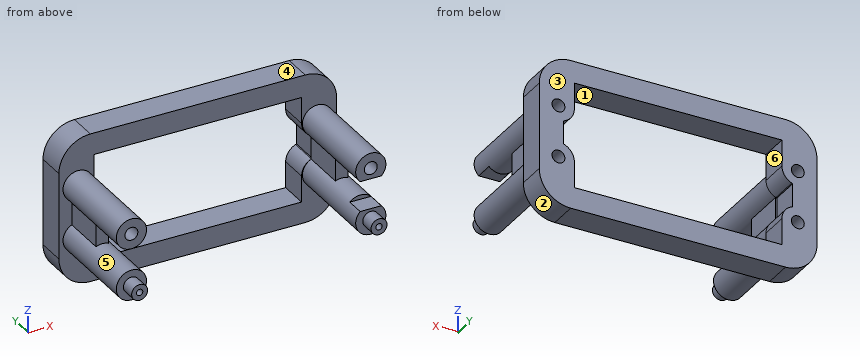
from build123d import *

# Parameters (mm, degrees)
SKETCH1_R           = 3.048
SKETCH1_R_2         = 1.2319
BOSS_EXTRUDE1_DEPTH = 25.4
SKETCH2_W           = 56.0832
SKETCH2_H           = 30.1244
BOSS_EXTRUDE3_DEPTH = 5.842
FILLET1_R           = 3.175
FILLET3_R           = 6.35
SKETCH6_W           = 5.842
SKETCH6_H           = 8.89
BOSS_EXTRUDE4_DEPTH = 1.27
SKETCH7_W           = 5.842
SKETCH7_H           = 8.89
BOSS_EXTRUDE5_DEPTH = 1.27
SKETCH16_R          = 1.6129
BOSS_EXTRUDE6_DEPTH = 3.0226
SKETCH19_R          = 1.30175
CUT_EXTRUDE1_DEPTH  = 63.809652383
SKETCH20_R          = 1.30175
CUT_EXTRUDE2_DEPTH  = 63.809652383
BOSS_EXTRUDE7_START = -12.3825
SKETCH21_R          = 1.30175
SKETCH21_R_2        = 0.635
BOSS_EXTRUDE7_DEPTH = 12.3825
SKETCH24_W          = 6.93711536
SKETCH24_H          = 6.096
CUT_EXTRUDE4_DEPTH  = 3.81


with BuildPart() as part:
    # Sketch1 → Boss-Extrude1 (new body)
    # profile 1 of 8: a face of its own
    with BuildSketch(Plane(origin=(0, 0, 0), x_dir=(1, 0, 0), z_dir=(0, 1, 0))):
        with Locations(Location((0, -10.4394, 0), (0, 0, 270))):
            Circle(SKETCH1_R)
        with Locations((0, -10.4394)):
            Circle(SKETCH1_R_2, mode=Mode.SUBTRACT)
    # profile 2 of 8: a face of its own
    with BuildSketch(Plane(origin=(0, 0, 0), x_dir=(1, 0, 0), z_dir=(0, 1, 0))):
        with Locations((0, -10.4394)):
            Circle(SKETCH1_R_2)
    # profile 3 of 8: a face of its own
    with BuildSketch(Plane(origin=(0, 0, 0), x_dir=(1, 0, 0), z_dir=(0, 1, 0))):
        with Locations(Location((0, 0, 0), (0, 0, 270))):
            Circle(SKETCH1_R)
        Circle(SKETCH1_R_2, mode=Mode.SUBTRACT)
    # profile 4 of 8: a face of its own
    with BuildSketch(Plane(origin=(0, 0, 0), x_dir=(1, 0, 0), z_dir=(0, 1, 0))):
        Circle(SKETCH1_R_2)
    # profile 5 of 8: a face of its own
    with BuildSketch(Plane(origin=(0, 0, 0), x_dir=(1, 0, 0), z_dir=(0, 1, 0))):
        with Locations(Location((-48.3362, -10.4394, 0), (0, 0, 270))):
            Circle(SKETCH1_R)
        with Locations((-48.3362, -10.4394)):
            Circle(SKETCH1_R_2, mode=Mode.SUBTRACT)
    # profile 6 of 8: a face of its own
    with BuildSketch(Plane(origin=(0, 0, 0), x_dir=(1, 0, 0), z_dir=(0, 1, 0))):
        with Locations((-48.3362, -10.4394)):
            Circle(SKETCH1_R_2)
    # profile 7 of 8: a face of its own
    with BuildSketch(Plane(origin=(0, 0, 0), x_dir=(1, 0, 0), z_dir=(0, 1, 0))):
        with Locations(Location((-48.3362, 0, 0), (0, 0, 270))):
            Circle(SKETCH1_R)
        with Locations((-48.3362, 0)):
            Circle(SKETCH1_R_2, mode=Mode.SUBTRACT)
    # profile 8 of 8: a face of its own
    with BuildSketch(Plane(origin=(0, 0, 0), x_dir=(1, 0, 0), z_dir=(0, 1, 0))):
        with Locations((-48.3362, 0)):
            Circle(SKETCH1_R_2)
    extrude(amount=-BOSS_EXTRUDE1_DEPTH)

    # Sketch2 → Boss-Extrude3 (add)
    with BuildSketch(Plane(origin=(0, 0, 0), x_dir=(1, 0, 0), z_dir=(0, 1, 0))):
        with Locations((-24.1681, -5.2197)):
            Rectangle(SKETCH2_W, SKETCH2_H)
        Polygon((-47.3075, -2.794), (-45.1231, -2.794), (-45.1231, 5.4483), (-3.2131, 5.4483), (-3.2131, -2.794), (-1.0287, -2.794), (-1.0287, -7.6454), (-3.2131, -7.6454), (-3.2131, -15.8877), (-45.1231, -15.8877), (-45.1231, -7.6454), (-47.3075, -7.6454), align=None, mode=Mode.SUBTRACT)
    extrude(amount=-BOSS_EXTRUDE3_DEPTH)

    # Fillet1
    # the kernel refuses this fillet: 3.175 mm, written as the material it takes off along each edge
    with BuildSketch(Plane(origin=(-3.2131, 7.368907547, 7.6454), x_dir=(1, 0, 0), z_dir=(0, -1, 0)), Plane(origin=(-45.1231, 7.368907547, 2.794), x_dir=(-1, 0, 0), z_dir=(0, -1, 0))) as fillet1_piece_1:
        with BuildLine():
            CenterArc((3.175, 2.947563019), FILLET1_R, 180, 68.181567229)
            Line((0, 2.947563019), (-0.0635, 2.947563019))
            Line((-0.0635, 2.947563019), (-0.0635, 0))
            Line((-0.0635, 0), (0, -0.0635))
            ThreePointArc((0, -0.0635), (0.997479397, -0.0635), (1.971357969, -0.05895126))
            Line((1.971357969, -0.05895126), (1.994958793, 0))
        make_face()
    extrude(amount=20.579815094, mode=Mode.SUBTRACT)
    with BuildSketch(Plane(origin=(-3.2131, 7.368907547, 2.794), x_dir=(0, 0, -1), z_dir=(0, -1, 0)), Plane(origin=(-45.1231, 7.368907547, 7.6454), x_dir=(0, 0, 1), z_dir=(0, -1, 0))) as fillet1_piece_2:
        with BuildLine():
            CenterArc((2.947563019, 3.175), FILLET1_R, 201.818432771, 68.181567229)
            Line((0, 1.994958793), (-0.05895126, 1.971357969))
            ThreePointArc((-0.05895126, 1.971357969), (-0.0635, 0.997479397), (-0.0635, 0))
            Line((-0.0635, 0), (0, -0.0635))
            Line((0, -0.0635), (2.947563019, -0.0635))
            Line((2.947563019, -0.0635), (2.947563019, 0))
        make_face()
    extrude(amount=20.579815094, mode=Mode.SUBTRACT)

    # Fillet3
    fillet3_edges = [part.edges().sort_by_distance(p)[0] for p in [
        (3.8735, -2.921, -9.8425),
        (3.8735, -2.921, 20.2819),
        (-52.2097, -2.921, 20.2819),
        (-52.2097, -2.921, -9.8425),
    ]]
    fillet(fillet3_edges, radius=FILLET3_R)

    # Sketch6 → Boss-Extrude4 (add, symmetric)
    with BuildSketch(Plane(origin=(0, 0, 0), x_dir=(0, 0, -1), z_dir=(1, 0, 0))):
        with Locations((-5.2197, -10.287)):
            Rectangle(SKETCH6_W, SKETCH6_H)
    extrude(amount=BOSS_EXTRUDE4_DEPTH, both=True)

    # Sketch7 → Boss-Extrude5 (add, symmetric)
    with BuildSketch(Plane.ZY.offset(48.3362)):
        with Locations((5.2197, -10.287)):
            Rectangle(SKETCH7_W, SKETCH7_H)
    extrude(amount=BOSS_EXTRUDE5_DEPTH, both=True)

    # Sketch16 → Boss-Extrude6 (add)
    with BuildSketch(Plane.XZ.offset(25.4)):
        with Locations(Location((0, 0, 0), (0, 0, 90))):
            Circle(SKETCH16_R)
        with Locations(Location((-48.3362, 0, 0), (0, 0, 90))):
            Circle(SKETCH16_R)
    extrude(amount=BOSS_EXTRUDE6_DEPTH)

    # Sketch19 → Cut-Extrude1 (cut, through all)
    with BuildSketch(Plane(origin=(0, 0, 0), x_dir=(1, 0, 0), z_dir=(0, 1, 0))):
        with Locations(Location((-48.3362, -10.4394, 0), (0, 0, 270))):
            Circle(SKETCH19_R)
        with Locations(Location((0, -10.4394, 0), (0, 0, 270))):
            Circle(SKETCH19_R)
    extrude(amount=-CUT_EXTRUDE1_DEPTH, mode=Mode.SUBTRACT)

    # Sketch20 → Cut-Extrude2 (cut, through all)
    with BuildSketch(Plane(origin=(0, 0, 0), x_dir=(1, 0, 0), z_dir=(0, 1, 0))):
        with Locations(Location((0, 0, 0), (0, 0, 270))):
            Circle(SKETCH20_R)
        with Locations(Location((-48.3362, 0, 0), (0, 0, 270))):
            Circle(SKETCH20_R)
    extrude(amount=-CUT_EXTRUDE2_DEPTH, mode=Mode.SUBTRACT)

    # Sketch21 → Boss-Extrude7 (add)
    # profile 1 of 2: a face of its own
    with BuildSketch(Plane.XZ.offset(28.4226).offset(BOSS_EXTRUDE7_START)):
        with Locations(Location((-48.3362, 0, 0), (0, 0, 90))):
            Circle(SKETCH21_R)
        with Locations(Location((-48.3362, 0, 0), (0, 0, 270))):
            Circle(SKETCH21_R_2, mode=Mode.SUBTRACT)
    # profile 2 of 2: a face of its own
    with BuildSketch(Plane.XZ.offset(28.4226).offset(BOSS_EXTRUDE7_START)):
        with Locations(Location((0, 0, 0), (0, 0, 90))):
            Circle(SKETCH21_R)
        with Locations(Location((0, 0, 0), (0, 0, 270))):
            Circle(SKETCH21_R_2, mode=Mode.SUBTRACT)
    extrude(amount=BOSS_EXTRUDE7_DEPTH)

    # Sketch24 → Cut-Extrude4 (cut)
    with BuildSketch(Plane.XZ.offset(25.4)):
        with Locations((0, 5.2197)):
            Rectangle(SKETCH24_W, SKETCH24_H)
    extrude(amount=-CUT_EXTRUDE4_DEPTH, mode=Mode.SUBTRACT)


solid = part.part
Geometry: final body of the model. Coordinates: model frame, mm. Face numbers are marked on the shaded views. A direction names the side the tool comes from. Coordinates: 2 decimals unless noted, no trailing zeros. Loops run counter-clockwise (first coordinate to the right, second up) from the corner with the lowest first, then second, coordinate; pieces in that order, holes last. Notation, with made-up numbers: (-24, -34.5) - (29, -34.5) arc R28 ccw to (29, -10.5) - close; hole circle Ø9 at (30, 3). An arc over 180 degrees is marked (long way). Put each result on its own line as item: value. Start each with the question number.
Q1. Cut plane D-D, the plane y = -24.5. Return loops of the section in (x, z) (1 decimal), and give its area (3 significant figures).
Q2. Cut plane B-B, the plane y = -12.25. Return loops of the section in (x, z), and give its area (3 significant figures).
Q3. Cut plane C-C, the plane x = 0. Give the number of separate pieces and of enclosed holes in the cut face, and give its area (3 significant figures).
Q4. Pin query (flat end, axial travel): pin 1 Ø2 at (x, z) = (-7, 16) entering from -Y; pin 2 Ø4 at (y, z) = (-25, 1) entering from -X; pin 3 Ø3.5 at (x, z) = (0, 0) entering from -Y; pin 4 Ø3 at (x, y) = (-0.5, -23.5) entering from -Z. Return the tip coordinate at first contact, or that it passes through.
Q5. Pull-direction query (X, two-part tool) for the marked faces 1, 2 and 3; classes: released by +X, released by -X, zero draft, split by the parting line, or undercut.
Q6. Cut plane A-A, the plane x = -6. Return loops of the section in (y, z).
Q7. Set-up query: the marked faces 4, 5 and 6. Return all of +Z, -Z, +X, -X, +Y, -Y with unobstructed straight access to the full face (end or side cutting, diameter ignored); none if empty.
Q8. Line query: line 1 (X direction, y = -21.75, z = 0) (3 decimals); line 2 (X direction, y = -25.75, z = 0) (3 decimals); line 3 (X direction, y = -14, z = 13). Output: solid intervals per line, ascending.
Filled sheet:
1. outline: circle Ø6.1 at (-48.3, 0); circle Ø6.1 at (-48.3, 10.4); (-2.1, 2.2) arc R3 ccw (long way) to (2.1, 2.2) - close; (-2.1, 8.3) - (2.1, 8.3) arc R3 ccw (long way) to start; hole circle Ø2.6 at (-48.3, 10.4); hole circle Ø1.3 at (-48.3, 0); hole circle Ø2.6 at (0, 10.4); hole circle Ø1.3 at (0, 0)
1. area: 98.4 mm²
2. outline: (-49.61, 2.77) arc R3.05 ccw (long way) to (-47.07, 2.77) - (-47.07, 7.67) arc R3.05 ccw (long way) to (-49.61, 7.67) - close; (-1.27, 2.77) arc R3.05 ccw (long way) to (1.27, 2.77) - (1.27, 7.67) arc R3.05 ccw (long way) to (-1.27, 7.67) - close; hole circle Ø2.6 at (-48.34, 0); hole circle Ø2.6 at (-48.34, 10.44); hole circle Ø2.6 at (0, 0); hole circle Ø2.6 at (0, 10.44)
2. area: 118 mm²
3. separate pieces: 3
3. enclosed holes: 0
3. area: 327 mm²
4. pin 1: y = -5.84
4. pin 2: x = -51.38
4. pin 3: y = -28.42
4. pin 4: z = -3.05
5. face 1: undercut
5. face 2: released by +X
5. face 3: zero draft
6. outline: (-5.84, -9.84) - (0, -9.84) - (0, -5.45) - (-5.84, -5.45) - close; (-5.84, 15.89) - (0, 15.89) - (0, 20.28) - (-5.84, 20.28) - close
7. face 4: +Z, +X, -X, +Y, -Y
7. face 5: -Y
7. face 6: +Y, -Y
8. line 1: -51.384 to -48.971, -47.701 to -45.288, -3.048 to -0.635, 0.635 to 3.048
8. line 2: -49.949 to -48.971, -47.701 to -46.723, -1.613 to -0.635, 0.635 to 1.613
8. line 3: -49.99 to -46.68, -1.65 to 1.65
